```python
from build123d import *

# Parameters (mm, degrees)
F0_W     = 12.7
F0_H     = 762
F1_DEPTH = 12.7
F2_SIZE  = 10.16


with BuildPart() as f1:
    # F0 (on Top) → F1 (new body)
    with BuildSketch(Plane.XY):
        with Locations((-53.53354, 320.315027)):
            Rectangle(F0_W, F0_H)
    extrude(amount=F1_DEPTH)

    # F2
    f2_edges = [f1.edges().sort_by_distance(p)[0] for p in [
        (-59.88354, 320.315027, 12.7),
        (-47.18354, 320.315027, 0),
    ]]
    chamfer(f2_edges, length=F2_SIZE)


solid = f1.part
```
The model under review builds one solid part; all positions refer to its coordinate system, in mm. Give positions to 0.01 mm unless a question says otherwise; leave off trailing zeros. Write each loop counter-clockwise with the first axis right and the second up, starting at its lowest first coordinate (ties: lowest second). Pieces come first, ordered by that corner, then holes. Notation, with made-up numbers: (0, 88) - (28, 88) arc R6 ccw to (28, 93) - close; hole circle Ø2 at (63.25, -22). An arc over 180 degrees is marked (long way). Answer in a Markdown table with one row per item. Add a question column.
1. Wall thickness on line 1 along Z through (x, y) = (-51.75, 47.5); line 2 along X through (y, z) = (13, 5.5); line 3 along Z through (x, y) = (-54, 114.5): over which ranges is each line inside the solid? List them lowest first. Write a range as [from, to].
2. We need section A-A on y = 300. Write out the cut boundary in (x, z).
3. Draft analysis for pull direction Y (two halves, no side actions). For faces 1 (the flat face through (-54, 701.315, 6)), 2 (the flat face through (-54, -60.685, 6)), state which applies: +Y half, -Y half, draft (parallel to the pull), parting line (faces both ways), or undercut.
4. We need section B-B on z = 7. Write out the cut boundary in (x, y), then the cut area to 3 significant figures.
5. Insertion check: P1, Ø3, axis at y = 465.5, z = 1.5, coming from the +X side; P2, Ø3, axis at x = -51.5, y = 199.5, coming from the +Z side. Each pin has a flat end and moves straight along its axis. Give the tip position at first contact, or say it passes through.
Ans:
| question | item | result |
|---|---|---|
| 1 | line 1 | z = [5.59, 10.67] |
| 1 | line 2 | x = [-56.92, -51.84] |
| 1 | line 3 | z = [3.34, 8.42] |
| 2 | outline | (-59.88, 0) - (-57.34, 0) - (-47.18, 10.16) - (-47.18, 12.7) - (-49.72, 12.7) - (-59.88, 2.54) - close |
| 3 | face 1 | +Y half |
| 3 | face 2 | -Y half |
| 4 | outline | (-55.42, -60.68) - (-50.34, -60.68) - (-50.34, 701.32) - (-55.42, 701.32) - close |
| 4 | area | 3,870 mm^2 |
| 5 | P1 | stops at x = -54.34 |
| 5 | P2 | stops at z = 12.42 |
